Work out the finished part from the listing and answer in its coordinate system (mm). A direction names the side the tool comes from. Round coordinates to 2 decimals unless told otherwise and drop trailing zeros. Write each loop counter-clockwise with the first axis right and the second up, starting at its lowest first coordinate (ties: lowest second). Pieces come first, ordered by that corner, then holes. Notation, with made-up numbers: M -30.5,84 L 6.5,84 A8 ccw 6.5,93 Z; hole C 76,-36 d1. An arc over 180 degrees is marked long. One line per item, written item: value. Start each with the question number.
Q1. Given pin 1 Ø9 at (x, z) = (-165, -60) entering from +Y; pin 2 Ø1 at (y, z) = (-25, -12.5) entering from -X; pin 3 Ø8 at (x, z) = (-120, -30) entering from -Y, each flat-ended and moving along its own axis, determine where each tip first touches the part or whether it passes through.
Q2. Find section C-C (x = -165). Write down the section's boundary in (y, z).
Q3. Consider probe 1 along Z at (x, y) = (-165, -57.9); probe 2 along X at (y, z) = (-46, -109); probe 3 along X at (y, z) = (-58.1, -60). Determine where each line is inside the solid, lowest interval first.
Q4. A tool of negligible diameter and unlimited length cuts with its end or side. For faces 4 (the flat face through (-150, -28, -59)), 5 (the flat face through (20, -56.94, -59)), 6 (the flat face through (-76, -3, -59)), from which of +Z, -Z, +X, -X, +Y, -Y can it reach the whole face along a straight path? Write none if from no direction.
Q5. Find section B-B (y = -33). Write down the section's boundary in (x, z), and give its area (3 significant figures).
Q6. Find section D-D (z = -60). Write down the section's boundary in (x, y), and give its area (3 significant figures).
Q7. The mould has two halves that part along Z. Classify faces 1 (the flat face through (-75, -1, -120)), 2 (the cylindrical face through (-167.1, -58.4, -62.8)), 3 (the cylindrical face through (-144.15, -6.01, -60.84)): released by +Z, released by -Z, zero draft, split by the parting line, or undercut.
Q8. Find section A-A (x = -120). Write down the section's boundary in (y, z), and give its area (3 significant figures).
from build123d import *

# Parameters (mm, degrees)
EXTRUDE_THIN1_DEPTH = 120
SKETCH2_R           = 3.5
CUT_EXTRUDE1_DEPTH  = 10
LPATTERN1_COUNT     = 2
LPATTERN1_PITCH     = 180
SKETCH3_R           = 3.5
CUT_EXTRUDE2_DEPTH  = 10
FILLET1_R           = 10


with BuildPart() as part:
    # Sketch1 → Extrude-Thin1 (new body)
    with BuildSketch(Plane.XY):
        Polygon((30, -56.94), (0, -56.94), (0, 0), (-150, 0), (-150, -56.94), (-180, -56.94), (-180, -59.94), (-147, -59.94), (-147, -3), (-3, -3), (-3, -59.94), (30, -59.94), align=None)
    extrude(amount=-EXTRUDE_THIN1_DEPTH)

    # Sketch2 → Cut-Extrude1 (cut)
    with BuildSketch(Plane(origin=(0, -56.94, 0), x_dir=(1, 0, 0), z_dir=(0, 1, 0))):
        with Locations(Location((15, 30, 0), (0, 0, 270))):
            Circle(SKETCH2_R)
        with Locations(Location((15, 60, 0), (0, 0, 270))):
            Circle(SKETCH2_R)
        with Locations(Location((15, 90, 0), (0, 0, 270))):
            Circle(SKETCH2_R)
    cut_extrude1 = extrude(amount=-CUT_EXTRUDE1_DEPTH, mode=Mode.SUBTRACT)

    # LPattern1: Cut-Extrude1 ×2
    with Locations(*[(-i * LPATTERN1_PITCH, 0, 0) for i in range(1, LPATTERN1_COUNT)]):
        add(cut_extrude1, mode=Mode.SUBTRACT)

    # Sketch3 → Cut-Extrude2 (cut)
    with BuildSketch(Plane(origin=(0, 0, 0), x_dir=(1, 0, 0), z_dir=(0, 1, 0))):
        with Locations(Location((-30, 30, 0), (0, 0, 270))):
            Circle(SKETCH3_R)
        with Locations(Location((-120, 30, 0), (0, 0, 270))):
            Circle(SKETCH3_R)
    extrude(amount=-CUT_EXTRUDE2_DEPTH, mode=Mode.SUBTRACT)

    # Fillet1
    fillet1_edges = [part.edges().sort_by_distance(p)[0] for p in [
        (-150, -56.94, -60),
        (-150, 0, -60),
        (0, 0, -60),
        (0, -56.94, -60),
        (-3, -59.94, -60),
        (-3, -3, -60),
        (-147, -3, -60),
        (-147, -59.94, -60),
    ]]
    fillet(fillet1_edges, radius=FILLET1_R)


solid = part.part
The answers:
1. pin 1: y = -56.94
1. pin 2: x = -150
1. pin 3: y = -3
2. outline: M -59.94,-120 L -56.94,-120 L -56.94,-93.5 L -59.94,-93.5 Z; M -59.94,-86.5 L -56.94,-86.5 L -56.94,-63.5 L -59.94,-63.5 Z; M -59.94,-56.5 L -56.94,-56.5 L -56.94,-33.5 L -59.94,-33.5 Z; M -59.94,-26.5 L -56.94,-26.5 L -56.94,0 L -59.94,0 Z
3. probe 1: -120 to -93.5, -86.5 to -63.5, -56.5 to -33.5, -26.5 to 0
3. probe 2: -150 to -147, -3 to 0
3. probe 3: -180 to -168.5, -161.5 to -151.22, 1.22 to 11.5, 18.5 to 30
4. face 4: +Z, -Z, -X, +Y
4. face 5: +Z, -Z, +X, +Y
4. face 6: +Z, -Z, -Y
5. outline: M -150,-120 L -147,-120 L -147,0 L -150,0 Z; M -3,-120 L 0,-120 L 0,0 L -3,0 Z
5. area: 720 mm2
6. outline: M -180,-59.94 L -168.5,-59.94 L -168.5,-56.94 L -180,-56.94 Z; M -161.5,-59.94 L -157,-59.94 A10 ccw -147,-49.94 L -147,-13 A10 cw -137,-3 L -13,-3 A10 cw -3,-13 L -3,-49.94 A10 ccw 7,-59.94 L 11.5,-59.94 L 11.5,-56.94 L 10,-56.94 A10 cw 0,-46.94 L 0,-10 A10 ccw -10,0 L -140,0 A10 ccw -150,-10 L -150,-46.94 A10 cw -160,-56.94 L -161.5,-56.94 Z; M 18.5,-59.94 L 30,-59.94 L 30,-56.94 L 18.5,-56.94 Z
6. area: 930 mm2
7. face 1: released by -Z
7. face 2: undercut
7. face 3: zero draft
8. outline: M -3,-120 L 0,-120 L 0,-33.5 L -3,-33.5 Z; M -3,-26.5 L 0,-26.5 L 0,0 L -3,0 Z
8. area: 339 mm2
